Geometry: final body of the model. Coordinates: model frame, mm. A direction names the side the tool comes from. Round coordinates to 2 decimals unless told otherwise and drop trailing zeros. Loops run counter-clockwise (first coordinate to the right, second up) from the corner with the lowest first, then second, coordinate; pieces in that order, holes last. Notation, with made-up numbers: (-32, 51.25) - (-20, 51.25) arc R19 ccw to (-20, 57.25) - close; hole circle Ø2 at (66.25, 86). An arc over 180 degrees is marked (long way). Answer as CSV lines item,"result".
from build123d import *

# Parameters (mm, degrees)
SKETCH1_R                = 20
BOSS_EXTRUDE1_DEPTH      = 3
SKETCH2_R                = 9
BOSS_EXTRUDE2_DEPTH      = 8
SKETCH4_R                = 6.35
CUT_EXTRUDE1_DEPTH       = 31.347981811
M3_TAPPED_HOLE1_REACH    = 37.917
M3_TAPPED_HOLE1_BORE_R   = 1.25
F_5_0_5_DIAMETER_HOLE1_D = 5
CIRPATTERN1_COUNT        = 4


with BuildPart() as part:
    # Sketch1 → Boss-Extrude1 (new body)
    with BuildSketch(Plane.XY):
        Circle(SKETCH1_R)
    extrude(amount=BOSS_EXTRUDE1_DEPTH)

    # Sketch2 → Boss-Extrude2 (add)
    with BuildSketch(Plane.XY.offset(3)):
        Circle(SKETCH2_R)
    extrude(amount=BOSS_EXTRUDE2_DEPTH)

    # Sketch4 → Cut-Extrude1 (cut, through all)
    with BuildSketch(Plane.XY.offset(11)):
        Circle(SKETCH4_R)
    extrude(amount=-CUT_EXTRUDE1_DEPTH, mode=Mode.SUBTRACT)

    # M3 Tapped Hole1 bore (on position points) → M3 Tapped Hole1 (cut, up to next)
    with BuildSketch(Plane(origin=(0, 9, 7), x_dir=(1, 0, 0), z_dir=(0, 1, 0)), mode=Mode.PRIVATE) as m3_tapped_hole1_sk1:
        Circle(M3_TAPPED_HOLE1_BORE_R)
    m3_tapped_hole1_tool1 = extrude(m3_tapped_hole1_sk1.sketch, amount=-M3_TAPPED_HOLE1_REACH, mode=Mode.PRIVATE) & part.part
    add(m3_tapped_hole1_tool1.solids().sort_by_distance((0, 9, 7))[0], mode=Mode.SUBTRACT)

    # Ø5.0 (5) Diameter Hole1 (through all)
    with Locations(Plane(origin=(11, 11, 3), x_dir=(1, 0, 0), z_dir=(0, 0, 1))):
        with Locations((0, 0)):
            f_5_0_5_diameter_hole1 = Hole(F_5_0_5_DIAMETER_HOLE1_D / 2)

    # CirPattern1: Ø5.0 (5) Diameter Hole1 ×4 about axis
    cirpattern1_axis = Axis((0, 0, 0), (0, 0, 1))
    for i in range(1, CIRPATTERN1_COUNT):
        add(f_5_0_5_diameter_hole1.rotate(cirpattern1_axis, i * 360 / CIRPATTERN1_COUNT), mode=Mode.SUBTRACT)


solid = part.part
(1) Draft query along Y for faces 1 (the face through (-4.336, -19.524, 1.479)), 2 (the face through (-8.56, 11.54, 1.48)), 3 (the face through (-11.54, -8.56, 1.48)), 4 (the face through (-5, 5, 0)). Return one class per face: pulls with the +Y half, pulls with the -Y half, needs draft (parallel to the pull), parting line crosses it, or undercut.
Findings below:
face 1,"parting line crosses it"
face 2,"undercut"
face 3,"undercut"
face 4,"needs draft"
(2) Section B-B (x = -11). Output: boundary loops of the cut face in (y, z).
Findings below:
outline,"(-16.7, 0) - (-13.5, 0) - (-13.5, 3) - (-16.7, 3) - close; (-8.5, 0) - (8.5, 0) - (8.5, 3) - (-8.5, 3) - close; (13.5, 0) - (16.7, 0) - (16.7, 3) - (13.5, 3) - close"
(3) Pin query (flat end, axial travel): P1, Ø3, axis at x = 2, z = 7.5, coming from the -Y side; P2, Ø1, axis at x = -7.5, z = 6, coming from the +Y side; P3, Ø4, axis at x = 11, y = -11, coming from the -Z side; P4, Ø6, axis at x = -11, y = -11, coming from the -Z side. Return the tip coordinate at first contact, or that it passes through.
Findings below:
P1,"y = -8.99"
P2,"y = 5.66"
P3,"through"
P4,"z = 0"
(4) Material intervals for line 1 along Z through (x, y) = (0, 8); line 2 along Z through (x, y) = (-12.5, -0.5); line 3 along Y through (x, z) = (0, 4.75), sorted ascending.
Findings below:
line 1,"0 to 5.75, 8.25 to 11"
line 2,"0 to 3"
line 3,"-9 to -6.35, 6.35 to 9"
(5) Section A-A (y = 0). Output: boundary loops of the cut face in (x, z), and give its area (3 significant figures).
Findings below:
outline,"(-20, 0) - (-6.35, 0) - (-6.35, 11) - (-9, 11) - (-9, 3) - (-20, 3) - close; (6.35, 0) - (20, 0) - (20, 3) - (9, 3) - (9, 11) - (6.35, 11) - close"
area,"124 mm2"
(6) Section C-C (x = -4.5). Output: boundary loops of the cut face in (y, z).
Findings below:
outline,"(-19.49, 0) - (-4.48, 0) - (-4.48, 11) - (-7.79, 11) - (-7.79, 3) - (-19.49, 3) - close; (4.48, 0) - (19.49, 0) - (19.49, 3) - (7.79, 3) - (7.79, 11) - (4.48, 11) - close"
(7) Access query for faces 5 (the face through (-1.951, -8.786, 6.944)), 6 (the face through (-0.27, 7.63, 8.22)), 7 (the face through (-1.38, -6.2, 5.58)). Directions: +Z, -Z, +X, -X, +Y, -Y. A direction counts if a zero-diameter tool reaches every point of the face in a straight line with its end or side. Return the directions, or none.
Findings below:
face 5,"+Z"
face 6,"+Y"
face 7,"+Z, -Z"
